```python
from build123d import *

# Parameters (mm, degrees)
F0_W      = 200.3522217274
F0_H      = 200.7694281638
F1_DEPTH  = 220
F2_W      = 106.5517105162
F2_H      = 12.7497781068
F3_DEPTH  = 15
F4_R      = 5
F5_R      = 5
F6_R      = 5
F8_R      = 5
F9_R      = 5
F12_DEPTH = 6.66
F14_R     = 8.8266857578
F14_R_2   = 8.8654347792
F14_R_3   = 9.3130675206
F14_R_4   = 9.3531300043
F15_DEPTH = 7
F7_R      = 11.1504231151
F18_DEPTH = 2


# Not quite as in the source:
# - the program builds the solid bodies; features that only make, move or delete a surface that nothing else refers to are left out


with BuildPart() as f1:
    # F0 (on Front) → F1 (new body)
    with BuildSketch(Plane.XZ):
        with Locations((35.5218797922, -56.1928581446)):
            Rectangle(F0_W, F0_H)
    extrude(amount=F1_DEPTH)

    # F2 (on face) → F3 (join)
    with BuildSketch(Plane.XZ.offset(220)):
        with Locations((33.8400062174, 20.9869192913)):
            Rectangle(F2_W, F2_H)
    extrude(amount=-F3_DEPTH)

    # F4
    f4_edges = [f1.edges().sort_by_distance(p)[0] for p in [
        (35.52188, -220, 44.191856),
    ]]
    fillet(f4_edges, radius=F4_R)

    # F5
    f5_edges = [f1.edges().sort_by_distance(p)[0] for p in [
        (135.697991, -218.535534, 42.72739),
    ]]
    fillet(f5_edges, radius=F5_R)

    # F6
    f6_edges = [f1.edges().sort_by_distance(p)[0] for p in [
        (-64.654231, -218.535534, 42.72739),
    ]]
    fillet(f6_edges, radius=F6_R)

    # F8
    f8_edges = [f1.edges().sort_by_distance(p)[0] for p in [
        (135.697991, -107.5, -156.577572),
        (35.52188, -220, -156.577572),
        (-64.654231, -107.5, -156.577572),
    ]]
    fillet(f8_edges, radius=F8_R)

    # F9
    f9_edges = [f1.edges().sort_by_distance(p)[0] for p in [
        (35.52188, 0, -156.577572),
    ]]
    fillet(f9_edges, radius=F9_R)

    # F2 (on face) → F12 (join)
    with BuildSketch(Plane.XZ.offset(220)):
        with Locations((33.8400062174, 20.9869192913)):
            Rectangle(F2_W, F2_H)
    extrude(amount=-F12_DEPTH)

    # F14 (on face) → F15 (join)
    with BuildSketch(Plane(origin=(0, 0, -156.5775722265), x_dir=(1, 0, 0), z_dir=(0, 0, -1))):
        with Locations((105.7562977076, 196.8253701925)):
            Circle(F14_R)
        with Locations((105.7562977076, 19.2491486669)):
            Circle(F14_R_2)
        with Locations((-43.5114949942, 20.4882938415)):
            Circle(F14_R_3)
        with Locations((-43.5114949942, 196.0519701242)):
            Circle(F14_R_4)
    extrude(amount=F15_DEPTH)

    # F7 (on face) → F18 (join)
    with BuildSketch(Plane(origin=(-64.6542310715, 0, 0), x_dir=(0, -1, 0), z_dir=(-1, 0, 0))):
        with Locations((199.0269720554, 21.7568427324)):
            Circle(F7_R)
    extrude(amount=F18_DEPTH)


solid = f1.part
```
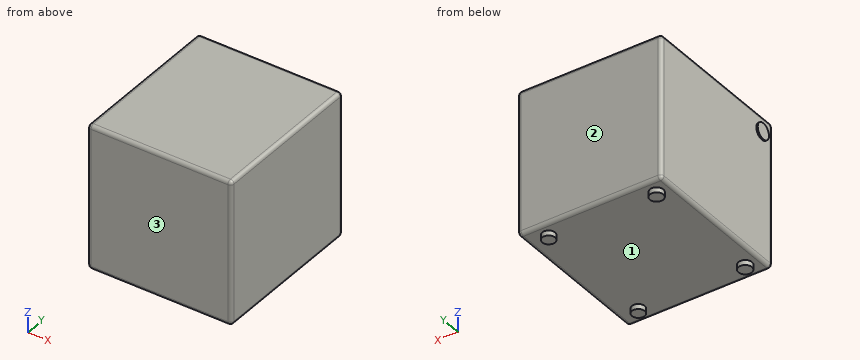
Could you check a few things on this model? Use its own coordinates, in mm. Face numbers are marked on the shaded views. Give positions to 0.01 mm unless a question says otherwise; leave off trailing zeros. Write each loop counter-clockwise with the first axis right and the second up, starting at its lowest first coordinate (ties: lowest second). Pieces come first, ordered by that corner, then holes. Notation, with made-up numbers: (70.5, 12.25) - (98.5, 12.25) arc R26 cw to (98.5, 49.25) - close; hole circle Ø9 at (60, -36.5). An arc over 180 degrees is marked (long way). One line per item, written item: value. Start each with the question number.
Item 1: Imagine slicing it at B-B, the plane y = -98. List the corners of the cut face in (x, z) for me, and give its area (3 significant figures).
Item 2: Please list where these lines run through material, in increasing order: line 1 (X direction, y = -22.5, z = -8); line 2 (Z direction, x = -56.5, y = -204); line 3 (X direction, y = -203, z = -155). Write a range as from..to.
Item 3: I'm going to push flat-ended pins straight in: pin 1 (12 mm diameter, centred on y = -85.5, z = -58.5, fed in from -X); pin 2 (4 mm diameter, centred on x = -13.5, y = -188, fed in from -Z). Where does each tip first touch, or does it pass through?
Item 4: If we mould it in two halves opening along Y, with no side actions, what happens to the marked faces 1, 2 and 3? For each: +Y half, -Y half, draft (parallel to the pull), parting line (faces both ways), or undercut.
Item 5: Imagine slicing it at A-A, the plane x = -1. List the corners of the cut face in (y, z) for me.
Item 6: Imagine slicing it at C-C, the plane x = 106. List the corners of the cut face in (y, z) for me, and give its area (3 significant figures).
Geometry says:
1. outline: (-64.65, -151.58) arc R5 ccw to (-59.65, -156.58) - (130.7, -156.58) arc R5 ccw to (135.7, -151.58) - (135.7, 39.19) arc R5 ccw to (130.7, 44.19) - (-59.65, 44.19) arc R5 ccw to (-64.65, 39.19) - close
1. area: 40,200 mm^2
2. line 1: -64.65..135.7
2. line 2: -156.58..44.19
2. line 3: -63.3..134.34
3. pin 1: x = -64.65
3. pin 2: z = -156.58
4. face 1: undercut
4. face 2: +Y half
4. face 3: -Y half
5. outline: (-220, -151.58) arc R5 ccw to (-215, -156.58) - (-5, -156.58) arc R5 ccw to (0, -151.58) - (0, 39.19) arc R5 ccw to (-5, 44.19) - (-215, 44.19) arc R5 ccw to (-220, 39.19) - close
6. outline: (-220, -151.58) arc R5 ccw to (-215, -156.58) - (-205.65, -156.58) - (-205.65, -163.58) - (-188, -163.58) - (-188, -156.58) - (-28.11, -156.58) - (-28.11, -163.58) - (-10.39, -163.58) - (-10.39, -156.58) - (-5, -156.58) arc R5 ccw to (0, -151.58) - (0, 39.19) arc R5 ccw to (-5, 44.19) - (-215, 44.19) arc R5 ccw to (-220, 39.19) - close
6. area: 44,400 mm^2
